Build history of the part. All positions in model axes, mm. Coordinates: 2 decimals unless noted, no trailing zeros. Write each loop counter-clockwise with the first axis right and the second up, starting at its lowest first coordinate (ties: lowest second). Pieces come first, ordered by that corner, then holes.
```python
from build123d import *

# Parameters (mm, degrees)
F0_W     = 279.4
F0_H     = 25.4
F0_W_2   = 152.4
F1_DEPTH = 12.7
F2_R     = 3.175
F3_DEPTH = 12.7


with BuildPart() as f1:
    # F0 (on Front) → F1 (new body, symmetric)
    with BuildSketch(Plane.XZ):
        with Locations((139.7, -12.7)):
            Rectangle(F0_W, F0_H)
        Polygon((0, -25.4), (0, 0), (-25.4, 0), (-25.4, -76.2), (0, -76.2), align=None)
        Polygon((304.8, 0), (279.4, 0), (279.4, -25.4), (279.4, -203.2), (304.8, -203.2), (304.8, -177.8), align=None)
        with Locations((381, -190.5)):
            Rectangle(F0_W_2, F0_H)
        Polygon((457.2, 0), (457.2, -177.8), (457.2, -203.2), (482.6, -203.2), (482.6, 0), align=None)
    extrude(amount=F1_DEPTH, both=True)

    # F2 (on Front) → F3 (cut, symmetric)
    with BuildSketch(Plane.XZ):
        with Locations((469.9, -101.6)):
            Circle(F2_R)
        with Locations((469.9, -50.8)):
            Circle(F2_R)
        with Locations((469.9, -152.4)):
            Circle(F2_R)
        with Locations((292.1, -50.8)):
            Circle(F2_R)
    extrude(amount=F3_DEPTH, both=True, mode=Mode.SUBTRACT)


solid = f1.part
```
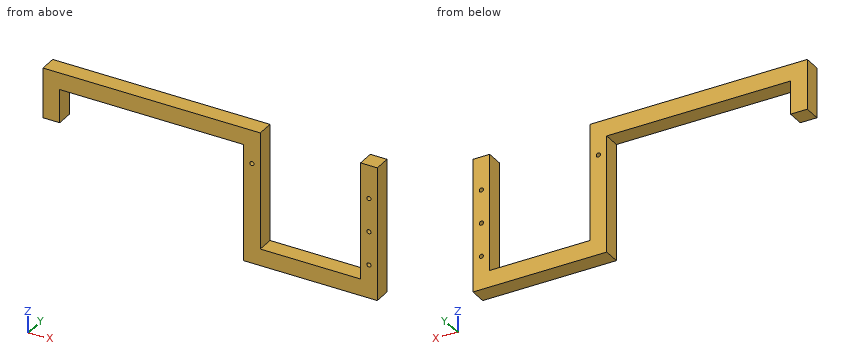
1. Saw through at B-B on y = 8.25. List the corners of the cut face in (x, z) (3 decimals).
Computed values:
outline: (-25.4, -76.2) - (0, -76.2) - (0, -25.4) - (279.4, -25.4) - (279.4, -203.2) - (482.6, -203.2) - (482.6, 0) - (457.2, 0) - (457.2, -177.8) - (304.8, -177.8) - (304.8, 0) - (-25.4, 0) - close; hole circle Ø6.35 at (292.1, -50.8); hole circle Ø6.35 at (469.9, -152.4); hole circle Ø6.35 at (469.9, -101.6); hole circle Ø6.35 at (469.9, -50.8)
2. Saw through at A-A on z = -68. List the corners of the cut face in (x, y), plus the area to 3 significant figures.
Computed values:
outline: (-25.4, -12.7) - (0, -12.7) - (0, 12.7) - (-25.4, 12.7) - close; (279.4, -12.7) - (304.8, -12.7) - (304.8, 12.7) - (279.4, 12.7) - close; (457.2, -12.7) - (482.6, -12.7) - (482.6, 12.7) - (457.2, 12.7) - close
area: 1,940 mm2
3. Flat gauge pin, fed straight in: pin 1 (2 mm diameter, centred on y = -9.5, z = -100, fed in from -X). Where does the tip first touch, or does it go through?
Computed values:
pin 1: stops at x = 279.4
4. Saw through at D-D on x = 17. List the corners of the cut face in (y, z).
Computed values:
outline: (-12.7, -25.4) - (12.7, -25.4) - (12.7, 0) - (-12.7, 0) - close
5. Probe line 1 along X through (y, z) = (8.25, -152.4) (3 decimals); line 2 along X through (y, z) = (-1.25, -74.5); line 3 along Z through (x, y) = (469.9, 7) (3 decimals). List the from-to ranges inside material, lowest first.
Computed values:
line 1: x = 279.4 to 304.8, 457.2 to 466.725, 473.075 to 482.6
line 2: x = -25.4 to 0, 279.4 to 304.8, 457.2 to 482.6
line 3: z = -203.2 to -155.575, -149.225 to -104.775, -98.425 to -53.975, -47.625 to 0
6. Saw through at C-C on z = -121. List the corners of the cut face in (x, y).
Computed values:
outline: (279.4, -12.7) - (304.8, -12.7) - (304.8, 12.7) - (279.4, 12.7) - close; (457.2, -12.7) - (482.6, -12.7) - (482.6, 12.7) - (457.2, 12.7) - close
